from build123d import *

# Parameters (mm, degrees)
CYLINDER048_R     = 5
CYLINDER048_DEPTH = 10
CYLINDER049_R     = 7.5
CYLINDER049_DEPTH = 5


with BuildPart() as cylinder048:
    # Cylinder048 → Cylinder048 (new body)
    with BuildSketch(Plane.XY):
        Circle(CYLINDER048_R)
    extrude(amount=CYLINDER048_DEPTH)


with BuildPart() as obj1:
    # Cylinder049 → Cylinder049 (new body)
    with BuildSketch(Plane.XY):
        Circle(CYLINDER049_R)
    extrude(amount=CYLINDER049_DEPTH)

    # Cut004037: cut Cylinder048
    add(cylinder048.part, mode=Mode.SUBTRACT)


solid = obj1.part
Verification items for the finished model (mm, model axes). Round coordinates to 2 decimals unless told otherwise and drop trailing zeros. Loops run counter-clockwise (first coordinate to the right, second up) from the corner with the lowest first, then second, coordinate; pieces in that order, holes last. Notation, with made-up numbers: (-19.75, 79) - (-0.75, 79) arc R18 cw to (-0.75, 90) - close; hole circle Ø1 at (1.5, 72.5). An arc over 180 degrees is marked (long way). Use a Markdown table: item, result. Add a question column.
1. Section check D-D, the plane x = -5.75. Record the boundary of the cut face in (y, z).
2. Thickness scan on probe 1 along Y at (x, z) = (0, 3.6); probe 2 along X at (y, z) = (1.25, 3.55); probe 3 along X at (y, z) = (3, 4.6). Record the ranges inside material, lowest first. Write a range as [from, to].
3. Section check A-A, the plane y = 0. Record the boundary of the cut face in (x, z).
4. Release check for a two-part mould opening along Y. For faces 1 (the face through (2, -5, 5)), 2 (the face through (-1.08, -4.88, 2.46)), 3 (the face through (-7.493, 0.33, 2.465)) record: released by +Y, released by -Y, zero draft, split by the parting line, or undercut.
5. Gauge pin test, flat ends, axial feed: pin 1 (3 mm diameter, centred on x = -2.5, z = 2.5, fed in from -Y); pin 2 (3 mm diameter, centred on x = 5.5, z = 1, fed in from +Y). Record the tip position at first contact, or that the pin passes through.
6. Section check C-C, the plane z = 4.05. Record the boundary of the cut face in (x, y), plus the area to 3 significant figures.
Checks:
| question | item | result |
|---|---|---|
| 1 | outline | (-4.82, 0) - (4.82, 0) - (4.82, 5) - (-4.82, 5) - close |
| 2 | probe 1 | y = [-7.5, -5], [5, 7.5] |
| 2 | probe 2 | x = [-7.4, -4.84], [4.84, 7.4] |
| 2 | probe 3 | x = [-6.87, -4], [4, 6.87] |
| 3 | outline | (-7.5, 0) - (-5, 0) - (-5, 5) - (-7.5, 5) - close; (5, 0) - (7.5, 0) - (7.5, 5) - (5, 5) - close |
| 4 | face 1 | zero draft |
| 4 | face 2 | undercut |
| 4 | face 3 | split by the parting line |
| 5 | pin 1 | stops at y = -7.43 |
| 5 | pin 2 | stops at y = 6.34 |
| 6 | outline | circle Ø15 at (0, 0); hole circle Ø10 at (0, 0) |
| 6 | area | 98.2 mm^2 |
